```python
from build123d import *

# Parameters (mm, degrees)
F0_W     = 100
F0_H     = 250
F1_DEPTH = 5
F3_R     = 2
F2_W     = 8
F2_H     = 230
F4_DEPTH = 25


with BuildPart() as f1:
    # F0 (on Top) → F1 (new body)
    with BuildSketch(Plane.XY):
        Rectangle(F0_W, F0_H)
    extrude(amount=F1_DEPTH)

    # F3
    f3_edges = [f1.edges().sort_by_distance(p)[0] for p in [
        (-50, 0, 0),
    ]]
    fillet(f3_edges, radius=F3_R)

    # F2 (on face) → F4 (cut)
    with BuildSketch(Plane.XY.offset(5)):
        with Locations((-35, 0)):
            Rectangle(F2_W, F2_H)
        with BuildLine():
            ThreePointArc((-31, 115), (-35, 119), (-39, 115))
            Line((-39, 115), (-31, 115))
        make_face()
        with BuildLine():
            Line((-31, -115), (-39, -115))
            ThreePointArc((-39, -115), (-35, -119), (-31, -115))
        make_face()
    extrude(amount=-F4_DEPTH, mode=Mode.SUBTRACT)


solid = f1.part
```
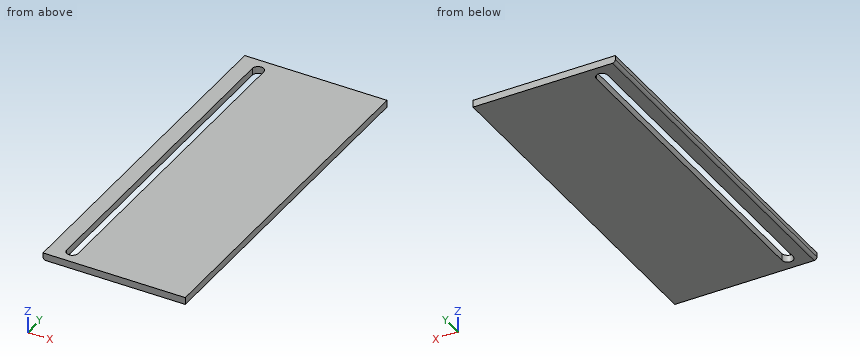
Check sheet for the modelled part. Datum: model origin and axes. Units: mm. Round coordinates to 2 decimals unless told otherwise and drop trailing zeros. Loops run counter-clockwise (first coordinate to the right, second up) from the corner with the lowest first, then second, coordinate; pieces in that order, holes last. Notation, with made-up numbers: (20.25, -14.75) - (59.25, -14.75) arc R22 ccw to (59.25, 21.25) - close; hole circle Ø5 at (60, 64). An arc over 180 degrees is marked (long way). Write item = value, one per line. Start each with the question number.
Q1. Section check A-A (x = -35). Record the boundary of the cut face in (y, z).
Q2. Thickness scan on L1, parallel to X at y = 42, z = 4.45; L2, parallel to X at y = 58.5, z = 0.2. Record the ranges inside material, lowest first.
Q3. Section check C-C (z = 0.9). Record the boundary of the cut face in (x, y).
Q4. Section check B-B (y = -4). Record the boundary of the cut face in (x, z), plus the area to 3 significant figures.
Derived:
q1.outline = (-125, 0) - (-119, 0) - (-119, 5) - (-125, 5) - close; (119, 0) - (125, 0) - (125, 5) - (119, 5) - close
q2.L1 = -50 to -39, -31 to 50
q2.L2 = -48.87 to -39, -31 to 50
q3.outline = (-49.67, -125) - (50, -125) - (50, 125) - (-49.67, 125) - close; hole (-39, -115) arc R4 ccw to (-31, -115) - (-31, 115) arc R4 ccw to (-39, 115) - close
q4.outline = (-50, 2) arc R2 ccw to (-48, 0) - (-39, 0) - (-39, 5) - (-50, 5) - close; (-31, 0) - (50, 0) - (50, 5) - (-31, 5) - close
q4.area = 459 mm^2
